Read the model definition and answer for the solid it produces. Units are mm, in the model's axes. Face numbers are marked on the shaded views. A direction names the side the tool comes from. Coordinates: 2 decimals unless noted, no trailing zeros. Write each loop counter-clockwise with the first axis right and the second up, starting at its lowest first coordinate (ties: lowest second). Pieces come first, ordered by that corner, then holes. Notation, with made-up numbers: (77.25, 60) -> (94.25, 60) arc R25 ccw to (94.25, 74) -> close; hole circle Ø8 at (62.25, 25.5). An arc over 180 degrees is marked (long way). Return JSON: item names as keys, results as strings.
from build123d import *

# Parameters (mm, degrees)
EXTRUDE_1_DEPTH     = 20
CUT_EXTRUDE_1_DEPTH = 82


with BuildPart() as part:
    # Эскиз1 → Бобышка-Вытянуть1 (new body)
    with BuildSketch(Plane.XY):
        with BuildLine():
            Line((0, 1), (0, 21))
            ThreePointArc((0, 21), (0.292893219, 21.707106781), (1, 22))
            Line((1, 22), (12.229943888, 22))
            ThreePointArc((12.229943888, 22), (12.937050669, 21.707106781), (13.229943888, 21))
            Line((13.229943888, 21), (13.229943888, 7))
            Line((13.229943888, 7), (41.229943888, 7))
            Line((41.229943888, 7), (68.26571085, 7))
            ThreePointArc((68.26571085, 7), (68.972817632, 6.707106781), (69.26571085, 6))
            Line((69.26571085, 6), (69.26571085, -19))
            ThreePointArc((69.26571085, -19), (68.972817632, -19.707106781), (68.26571085, -20))
            Line((68.26571085, -20), (63.26571085, -20))
            ThreePointArc((63.26571085, -20), (62.558604069, -19.707106781), (62.26571085, -19))
            Line((62.26571085, -19), (62.26571085, -1))
            ThreePointArc((62.26571085, -1), (61.972817632, -0.292893219), (61.26571085, 0))
            Line((61.26571085, 0), (51.26571085, 0))
            ThreePointArc((51.26571085, 0), (50.558604069, -0.292893219), (50.26571085, -1))
            Line((50.26571085, -1), (50.26571085, -19))
            ThreePointArc((50.26571085, -19), (49.972817632, -19.707106781), (49.26571085, -20))
            Line((49.26571085, -20), (44.26571085, -20))
            ThreePointArc((44.26571085, -20), (43.558604069, -19.707106781), (43.26571085, -19))
            Line((43.26571085, -19), (43.26571085, 0))
            Line((43.26571085, 0), (1, 0))
            ThreePointArc((1, 0), (0.292893219, 0.292893219), (0, 1))
        make_face()
    extrude(amount=EXTRUDE_1_DEPTH)

    # Эскиз2 → Вырез-Вытянуть1 (cut)
    with BuildSketch(Plane(origin=(0, 22, 0), x_dir=(1, 0, 0), z_dir=(0, 1, 0))):
        Polygon((81.392917707, -5), (0, 0), (88.471949447, 13.866629824), align=None)
        Polygon((81.392917707, -15), (0, -20), (97.493424041, -39.682856986), align=None)
    extrude(amount=-CUT_EXTRUDE_1_DEPTH, mode=Mode.SUBTRACT)


solid = part.part
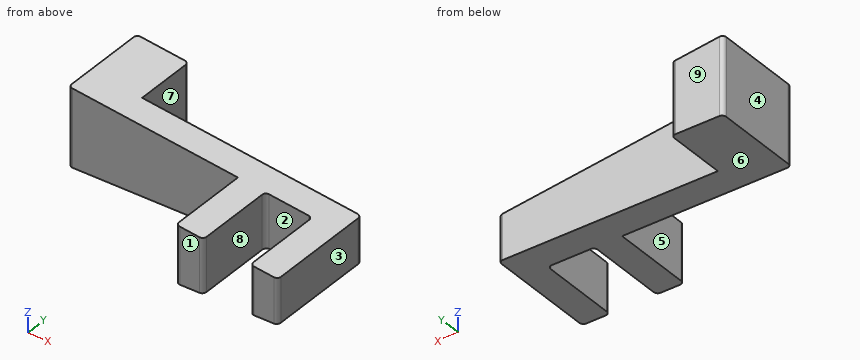
1. A tool of negligible diameter and unlimited length cuts with its end or side. For the marked faces 5, 6, 7, 8 and 9, from which of +Z, -Z, +X, -X, +Y, -Y can it reach the whole face along a straight path? Write none if from no direction.
Taken from the geometry:
{"face 5": "+Z, -Z, -X, -Y", "face 6": "-Z, +X, +Y, -Y", "face 7": "+Z, -Z, +X, +Y", "face 8": "+Z, -Z, -Y", "face 9": "+Z, -Z, +X, -X, +Y"}
2. The part is cut by section B-B (z = 8.5). Determine the outline of the cut face in (x, y), then the cut area to 3 significant figures.
Taken from the geometry:
{"outline": "(0, 1) arc R1 ccw to (1, 0) -> (43.27, 0) -> (43.27, -19) arc R1 ccw to (44.27, -20) -> (49.27, -20) arc R1 ccw to (50.27, -19) -> (50.27, -1) arc R1 cw to (51.27, 0) -> (61.27, 0) arc R1 cw to (62.27, -1) -> (62.27, -19) arc R1 ccw to (63.27, -20) -> (68.27, -20) arc R1 ccw to (69.27, -19) -> (69.27, 6) arc R1 ccw to (68.27, 7) -> (13.23, 7) -> (13.23, 21) arc R1 ccw to (12.23, 22) -> (1, 22) arc R1 ccw to (0, 21) -> close", "area": "962 mm2"}
3. The part is cut by section C-C (y = 10). Determine the outline of the cut face in (x, z), then the cut area to 3 significant figures.
Taken from the geometry:
{"outline": "(0, 0) -> (13.23, 0.81) -> (13.23, 19.19) -> (0, 20) -> close", "area": "254 mm2"}
4. The part is cut by section D-D (x = 39). Determine the outline of the cut face in (y, z), then the cut area to 3 significant figures.
Taken from the geometry:
{"outline": "(0, 2.4) -> (7, 2.4) -> (7, 17.6) -> (0, 17.6) -> close", "area": "106 mm2"}
5. Consider L1, parallel to X at y = 16.5, z = 15; L2, parallel to Y at x = 65, z = 6.5; L3, parallel to X at y = -5.5, z = 7. Determine where each line is inside the solid, lowest interval first.
Taken from the geometry:
{"L1": "x = 0 to 13.23", "L2": "y = -20 to 7", "L3": "x = 43.27 to 50.27, 62.27 to 69.27"}
6. The part is cut by section A-A (y = -4.5). Determine the outline of the cut face in (x, z) (3 decimals), then the cut area to 3 significant figures.
Taken from the geometry:
{"outline": "(43.266, 2.658) -> (50.266, 3.088) -> (50.266, 16.912) -> (43.266, 17.342) -> close; (62.266, 3.825) -> (69.266, 4.255) -> (69.266, 15.745) -> (62.266, 16.175) -> close", "area": "183 mm2"}
7. For a pull along X with two mould halves and no side action, classify the marked faces 1, 2, 3 and 4 as +X half, -X half, draft (parallel to the pull), parting line (faces both ways), or undercut.
Taken from the geometry:
{"face 1": "draft", "face 2": "undercut", "face 3": "+X half", "face 4": "-X half"}
8. Flat-ended cylindrical pins translate along their axes: pin 1 Ø4 at (x, z) = (21.5, 4) entering from +Y; pin 2 Ø4 at (y, z) = (-14.5, 10.5) entering from -X; pin 3 Ø10 at (x, y) = (50.5, -6.5) entering from +Z; pin 4 Ø10 at (x, y) = (37.5, -14.5) entering from -Z. Find the tip coordinate at first contact, or state that the pin passes through.
Taken from the geometry:
{"pin 1": "stops at y = 7", "pin 2": "stops at x = 43.27", "pin 3": "stops at z = 17.2", "pin 4": "passes through"}
